Build history of the part. All positions in model axes, mm. A direction names the side the tool comes from. Give positions to 0.01 mm unless a question says otherwise; leave off trailing zeros. Order: outer loops, then holes, each group sorted by start corner. A loop starts at its lowest first (then second) coordinate and runs counter-clockwise, first axis right, second up. Notation, with made-up numbers: M 44,64.5 L 88,64.5 A26 cw 88,97.5 Z; hole C 4,84 d10. An arc over 180 degrees is marked long. One line per item, written item: value.
from build123d import *

# Parameters (mm, degrees)
EXTRUDE_1_DEPTH          = 40
CUT_EXTRUDE_1_DEPTH      = 368
CUT_EXTRUDE_1_DEPTH_BACK = 39
SKETCH_2_R               = 19.5
CUT_EXTRUDE_2_DEPTH      = 39


with BuildPart() as part:
    # 草图1 → 凸台-拉伸1 (new body)
    with BuildSketch(Plane.XY):
        Polygon((-52.98729817, 27.74861141), (-52.98729817, -141.75138859), (231.01270183, -141.75138859), (231.01270183, 27.74861141), (229.51270183, 27.74861141), (229.51270183, -140.25138859), (-51.48729817, -140.25138859), (-51.48729817, 27.74861141), align=None)
    extrude(amount=EXTRUDE_1_DEPTH)

    # 草图2 → 切除-拉伸1 (cut, two sides: drawn at the far end of the back side and taken through both)
    with BuildSketch(Plane(origin=(-51.48729817, 0, 0), x_dir=(0, 0, -1), z_dir=(1, 0, 0)).offset(-CUT_EXTRUDE_1_DEPTH_BACK)):
        with Locations((-20, 27.74861141)):
            Circle(SKETCH_2_R)
    extrude(amount=CUT_EXTRUDE_1_DEPTH + CUT_EXTRUDE_1_DEPTH_BACK, mode=Mode.SUBTRACT)

    # 草图4 → 切除-拉伸2 (cut)
    with BuildSketch(Plane(origin=(0, -140.25138859, 0), x_dir=(1, 0, 0), z_dir=(0, 1, 0))):
        Polygon((89.01270183, -40), (53.81270183, -40), (53.81270183, -12), (89.01270183, -12), (124.21270183, -12), (124.21270183, -40), align=None)
    extrude(amount=-CUT_EXTRUDE_2_DEPTH, mode=Mode.SUBTRACT)


solid = part.part
1) Mould opens along Z. For faces 3 (the face through (-52.248, 8.253, 20.429)), 4 (the face through (87, -141.751, 11)), 5 (the face through (230.252, 8.253, 20.429)) say: released by +Z, released by -Z, zero draft, split by the parting line, or undercut.
Check values:
face 3: undercut
face 4: zero draft
face 5: undercut
2) Saw through at D-D, the plane z = 34. Write the cut outline in (x, y), then the cut area to 3 significant figures.
Check values:
outline: M -52.99,-141.75 L 53.81,-141.75 L 53.81,-140.25 L -51.49,-140.25 L -51.49,14.17 L -52.99,14.17 Z; M 124.21,-141.75 L 231.01,-141.75 L 231.01,14.17 L 229.51,14.17 L 229.51,-140.25 L 124.21,-140.25 Z
area: 784 mm^2
3) Saw through at A-A, the plane y = -104. Write the cut outline in (x, z), then the cut area to 3 significant figures.
Check values:
outline: M -52.99,0 L -51.49,0 L -51.49,40 L -52.99,40 Z; M 229.51,0 L 231.01,0 L 231.01,40 L 229.51,40 Z
area: 120 mm^2
4) Drill centre lines: probe 1 along X at (y, z) = (-47, 16); probe 2 along Y at (x, z) = (49, 23.5). Where is each one in solid material? Low to high. Write a range as from..to.
Check values:
probe 1: -52.99..-51.49, 229.51..231.01
probe 2: -141.75..-140.25
5) Saw through at C-C, the plane x = 176. Write the cut outline in (y, z).
Check values:
outline: M -141.75,0 L -140.25,0 L -140.25,40 L -141.75,40 Z
6) Saw through at B-B, the plane z = 20. Write the cut outline in (x, y).
Check values:
outline: M -52.99,-141.75 L 53.81,-141.75 L 53.81,-140.25 L -51.49,-140.25 L -51.49,8.25 L -52.99,8.25 Z; M 124.21,-141.75 L 231.01,-141.75 L 231.01,8.25 L 229.51,8.25 L 229.51,-140.25 L 124.21,-140.25 Z
7) Tool access for faces 1 (the face through (231.013, -58, 20)), 2 (the face through (91, -140.251, 11)): list every direction of +Z, -Z, +X, -X, +Y, -Y with a clear straight run to the whole face (end or side of a thin tool).
Check values:
face 1: +Z, -Z, +X, +Y, -Y
face 2: +Z, -Z, +Y
8) Pin check, flat tips, straight feed: pin 1 (20 mm diameter, centred on x = 149.5, z = 21.5, fed in from +Y); pin 2 (1.2 mm diameter, centred on x = 90, y = -141, fed in from +Z). Stop position of each tip, or through.
Check values:
pin 1: y = -140.25
pin 2: z = 12
